from build123d import *

# Parameters (mm, degrees)
F0_W     = 180
F0_H     = 150
F0_R     = 2.95
F1_DEPTH = 15
F2_DEPTH = 25
F3_SIZE  = 1
F4_SIZE  = 5


with BuildPart() as f1:
    # F0 (on Top) → F1 (new body)
    with BuildSketch(Plane.XY):
        Rectangle(F0_W, F0_H)
        Polygon((-30, 45), (30, 45), (30, 60), (70, 60), (70, -60), (30, -60), (30, -45), (-30, -45), (-30, -60), (-70, -60), (-70, 60), (-30, 60), align=None, mode=Mode.SUBTRACT)
        Polygon((-30, -45), (-30, 45), (-30, 60), (-70, 60), (-70, -60), (-30, -60), align=None)
        with Locations((-50, -44)):
            Circle(F0_R, mode=Mode.SUBTRACT)
        with Locations((-50, 44)):
            Circle(F0_R, mode=Mode.SUBTRACT)
        Polygon((30, 60), (30, 45), (30, -45), (30, -60), (70, -60), (70, 60), align=None)
        with Locations((50, -44)):
            Circle(F0_R, mode=Mode.SUBTRACT)
        with Locations((50, 44)):
            Circle(F0_R, mode=Mode.SUBTRACT)
    extrude(amount=-F1_DEPTH)

    # F0 (on Top) → F2 (join)
    with BuildSketch(Plane.XY):
        Polygon((-30, -45), (-30, 45), (-30, 60), (-70, 60), (-70, -60), (-30, -60), align=None)
        with Locations((-50, -44)):
            Circle(F0_R, mode=Mode.SUBTRACT)
        with Locations((-50, 44)):
            Circle(F0_R, mode=Mode.SUBTRACT)
        Polygon((30, 60), (30, 45), (30, -45), (30, -60), (70, -60), (70, 60), align=None)
        with Locations((50, -44)):
            Circle(F0_R, mode=Mode.SUBTRACT)
        with Locations((50, 44)):
            Circle(F0_R, mode=Mode.SUBTRACT)
    extrude(amount=F2_DEPTH)

    # F3
    f3_edges = [f1.edges().sort_by_distance(p)[0] for p in [
        (-70, -60, 12.5),
        (-30, -60, 12.5),
        (30, -60, 12.5),
        (70, -60, 12.5),
        (70, 60, 12.5),
        (30, 60, 12.5),
        (-30, 60, 12.5),
        (-70, 60, 12.5),
    ]]
    chamfer(f3_edges, length=F3_SIZE)

    # F4
    f4_edges = [f1.edges().sort_by_distance(p)[0] for p in [
        (0, 45, 0),
        (0, -45, 0),
        (-90, 0, 0),
        (90, 0, 0),
    ]]
    chamfer(f4_edges, length=F4_SIZE)


solid = f1.part
Design review of the part built by this model. Coordinates are the model's own, in mm. A direction names the side the tool comes from. Give positions to 0.01 mm unless a question says otherwise; leave off trailing zeros. Order: outer loops, then holes, each group sorted by start corner. A loop starts at its lowest first (then second) coordinate and runs counter-clockwise, first axis right, second up. Notation, with made-up numbers: (-39.75, 12.25) - (13.25, 12.25) arc R14 ccw to (13.25, 20.25) - close; hole circle Ø7 at (88.25, 1.5). An arc over 180 degrees is marked (long way). Write item = value, one per line. Start each with the question number.
Q1. We need section C-C on y = 29. State the section outline as (x, z) points.
Q2. Tool access review of faces 4 (the face through (30, 1, 5)), 5 (the face through (50, -60, 12)), 6 (the face through (0, -45, -10)): name each direction out of +Z, -Z, +X, -X, +Y, -Y from which nothing blocks a thin tool from reaching the whole face with its end or side.
Q3. Clearance check with flat-ended pins moving along their axes: pin 1 Ø7.5 at (x, z) = (48.5, 14.5) entering from +Y; pin 2 Ø12.5 at (x, z) = (-49, 15.5) entering from -Y; pin 3 Ø20 at (y, z) = (-29.5, 5.5) entering from +X. State where each tip first meets the part, or that it passes through.
Q4. We need section B-B on x = -50. State the section outline as (y, z) points.
Q5. Mouldability with a two-part tool opening along X and no side actions: class faces 1 (the face through (47.659, -45.795, 4.72)), 2 (the face through (-50, 60, 12)), 3 (the face through (70, -1, 12)) as released by +X, released by -X, zero draft, split by the parting line, or undercut.
Q6. To check wall thickness, follow L1, parallel to Y at x = 50, z = 7.5; L2, parallel to X at y = 34.5, z = 7; L3, parallel to Y at x = 50, z = -5. State the ranges of each line that lie inside material, in increasing order. Write a range as from..to.
Q7. We need section A-A on z = 14.5. State the section outline as (x, y) points.
Q8. We need section D-D on x = 13. State the section outline as (y, z) points, plus the area to 3 significant figures.
Working result:
q1.outline = (-90, -15) - (-30, -15) - (-30, 25) - (-70, 25) - (-70, 0) - (-85, 0) - (-90, -5) - close; (30, -15) - (90, -15) - (90, -5) - (85, 0) - (70, 0) - (70, 25) - (30, 25) - close
q2.face_4 = +Z
q2.face_5 = +Z, +X, -X, -Y
q2.face_6 = +Z, -Z
q3.pin_1 = 60
q3.pin_2 = -60
q3.pin_3 = 89.5
q4.outline = (-75, -15) - (-46.95, -15) - (-46.95, 25) - (-60, 25) - (-60, 0) - (-75, 0) - close; (-41.05, -15) - (41.05, -15) - (41.05, 25) - (-41.05, 25) - close; (46.95, -15) - (75, -15) - (75, 0) - (60, 0) - (60, 25) - (46.95, 25) - close
q5.face_1 = undercut
q5.face_2 = zero draft
q5.face_3 = released by +X
q6.L1 = -60..-46.95, -41.05..41.05, 46.95..60
q6.L2 = -70..-30, 30..70
q6.L3 = -75..-46.95, -41.05..41.05, 46.95..75
q7.outline = (-70, -59) - (-69, -60) - (-31, -60) - (-30, -59) - (-30, 59) - (-31, 60) - (-69, 60) - (-70, 59) - close; (30, -59) - (31, -60) - (69, -60) - (70, -59) - (70, 59) - (69, 60) - (31, 60) - (30, 59) - close; hole circle Ø5.9 at (-50, -44); hole circle Ø5.9 at (-50, 44); hole circle Ø5.9 at (50, -44); hole circle Ø5.9 at (50, 44)
q8.outline = (-75, -15) - (-45, -15) - (-45, -5) - (-50, 0) - (-75, 0) - close; (45, -15) - (75, -15) - (75, 0) - (50, 0) - (45, -5) - close
q8.area = 875 mm²
